Can you work these out from the model? Positions are in its coordinate system, mm. Face numbers are marked on the shaded views. Round coordinates to 2 decimals unless told otherwise and drop trailing zeros. Loops run counter-clockwise (first coordinate to the right, second up) from the corner with the lowest first, then second, coordinate; pieces in that order, holes last. Notation, with made-up numbers: (31.25, 12) -> (89.25, 12) arc R24 cw to (89.25, 48) -> close; hole circle Ø10 at (-11, 56). An arc over 180 degrees is marked (long way). Write item = value, one per line.
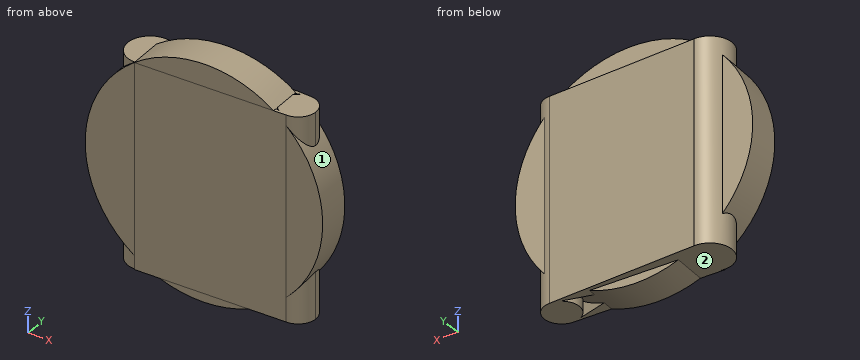
from build123d import *

# Parameters (mm, degrees)
F1_DEPTH = 152.4
F2_R     = 87.7285820259
F3_DEPTH = 25.4


with BuildPart() as f1:
    # F0 (on Top) → F1 (new body)
    with BuildSketch(Plane.XY):
        with BuildLine():
            ThreePointArc((4.3483612884, -16.0341400475), (13.1955019604, -10.0935930654), (16.6133046971, 0))
            ThreePointArc((16.6133046971, 0), (14.3717652499, 8.3339220395), (8.2520234436, 14.4189459408))
            Line((8.2520234436, 14.4189459408), (0, 16.6133046971))
            ThreePointArc((0, 16.6133046971), (-16.4678770205, -2.1933808143), (4.3483612884, -16.0341400475))
        make_face()
        with BuildLine():
            ThreePointArc((8.2520234436, 14.4189459408), (14.3717652499, 8.3339220395), (16.6133046971, 0))
            ThreePointArc((16.6133046971, 0), (13.1955019604, -10.0935930654), (4.3483612884, -16.0341400475))
            Line((4.3483612884, -16.0341400475), (62.9788908632, -0.1338945288))
            Line((62.9788908632, -0.1338945288), (8.2520234436, 14.4189459408))
        make_face()
        with BuildLine():
            Line((0, 16.6133046971), (8.2520234436, 14.4189459408))
            ThreePointArc((8.2520234436, 14.4189459408), (4.7563486134, 15.9178843075), (1.0113711573, 16.5824914093))
            Line((1.0113711573, 16.5824914093), (0, 16.6133046971))
        make_face()
        with BuildLine():
            ThreePointArc((1.0113711573, 16.5824914093), (4.7563486134, 15.9178843075), (8.2520234436, 14.4189459408))
            Line((8.2520234436, 14.4189459408), (62.9788908632, -0.1338945288))
            Line((62.9788908632, -0.1338945288), (105.4673896361, 11.3887297271))
            ThreePointArc((105.4673896361, 11.3887297271), (108.6807109667, 12.7368450388), (112.1348664165, 13.1969091614))
            Line((112.1348664165, 13.1969091614), (1.0113711573, 16.5824914093))
        make_face()
        with BuildLine():
            Line((62.9788908632, -0.1338945288), (4.3483612884, -16.0341400475))
            Line((4.3483612884, -16.0341400475), (0, -17.2133893668))
            Line((0, -17.2133893668), (112.1348664165, -13.2053364746))
            Line((112.1348664165, -13.2053364746), (112.1030305721, -13.1968707614))
            ThreePointArc((112.1030305721, -13.1968707614), (108.7434350674, -12.7536898511), (105.6074566347, -11.469582946))
            Line((105.6074566347, -11.469582946), (62.9788908632, -0.1338945288))
        make_face()
        with BuildLine():
            Line((0, 16.6133046971), (1.0113711573, 16.5824914093))
            ThreePointArc((1.0113711573, 16.5824914093), (0.5059202201, 16.6055995883), (0, 16.6133046971))
        make_face()
        with BuildLine():
            Line((105.4673896361, 11.3887297271), (112.1348664165, 13.1969091614))
            ThreePointArc((112.1348664165, 13.1969091614), (108.6807109667, 12.7368450388), (105.4673896361, 11.3887297271))
        make_face()
        with BuildLine():
            ThreePointArc((125.3317755778, 0), (121.4664903752, 9.3316239587), (112.1348664165, 13.1969091614))
            Line((112.1348664165, 13.1969091614), (105.4673896361, 11.3887297271))
            ThreePointArc((105.4673896361, 11.3887297271), (98.9382050049, -0.0808640945), (105.6074566347, -11.469582946))
            Line((105.6074566347, -11.469582946), (112.1030305721, -13.1968707614))
            ThreePointArc((112.1030305721, -13.1968707614), (121.455227908, -9.3428728494), (125.3317755778, 0))
        make_face()
        with BuildLine():
            Line((112.1030305721, -13.1968707614), (105.6074566347, -11.469582946))
            ThreePointArc((105.6074566347, -11.469582946), (108.7434350674, -12.7536898511), (112.1030305721, -13.1968707614))
        make_face()
    extrude(amount=F1_DEPTH)

    # F2 (on face) → F3 (join)
    with BuildSketch(Plane(origin=(0.6144756506, -17.1914260739, 0), x_dir=(0.9993618252, 0.0357203355, 0), z_dir=(0.0357203355, -0.9993618252, 0))):
        with Locations((50.8590377867, 81.3547074795)):
            Circle(F2_R)
    extrude(amount=-F3_DEPTH)


solid = f1.part
1. Suppose I cut it at A-A, the plane z = 100. List the corners of the cut face in (x, y) for me.
Entries:
outline = (-35.14, 6.95) -> (-34.23, -18.44) -> (137.11, -12.31) -> (136.2, 13.07) -> (116.72, 12.37) arc R13.2 ccw to (112.13, 13.2) -> (1.01, 16.58) arc R16.61 ccw to (-14.73, 7.68) -> close
2. I'm going to push flat-ended pins straight in: pin 1 (4 mm diameter, centred on x = 91, y = 1, fed in from +Z); pin 2 (5 mm diameter, centred on x = -16.5, y = 1, fed in from +Z); pin 3 (3 mm diameter, centred on y = 8.5, z = 74.5, fed in from +X). Where does each tip first touch, or does it pass through?
Entries:
pin_1 = 160.37
pin_2 = 152.4
pin_3 = 138.22
3. Suppose I cut it at B-B, the plane z = 75. List the corners of the cut face in (x, y) for me, and give its area (3 significant figures).
Entries:
outline = (-36.91, 6.88) -> (-36, -18.5) -> (138.88, -12.25) -> (137.98, 13.13) -> (116.72, 12.37) arc R13.2 ccw to (112.13, 13.2) -> (1.01, 16.58) arc R16.61 ccw to (-14.73, 7.68) -> close
area = 5,060 mm²
4. I need wall thicknesses on line 1 (Z direction, x = 107, y = -1); line 2 (X direction, y = 8.5, z = 6.5); line 3 (X direction, y = -12, z = 75). Which ranges of each line are inside material? Lowest first, please. Write a range as [from, to].
Entries:
line_1 = [0, 152.4]
line_2 = [-14.27, 96.37], [102.04, 122.23]
line_3 = [-36.23, 138.87]
5. Suppose I cut it at C-C, the plane z = 27.5. List the corners of the cut face in (x, y) for me, and give its area (3 significant figures).
Entries:
outline = (-18.68, 7.54) -> (-17.77, -17.85) -> (120.65, -12.9) -> (120.55, -10.16) arc R13.2 ccw to (119.8, 10.74) -> (119.74, 12.48) -> (116.72, 12.37) arc R13.2 ccw to (112.13, 13.2) -> (1.01, 16.58) arc R16.61 ccw to (-14.73, 7.68) -> close
area = 4,210 mm²
6. We'd pull the mould along X, two halves only. Please class the marked faces 1 and 2: released by +X, released by -X, zero draft, split by the parting line, or undercut.
Entries:
face_1 = released by +X
face_2 = zero draft
